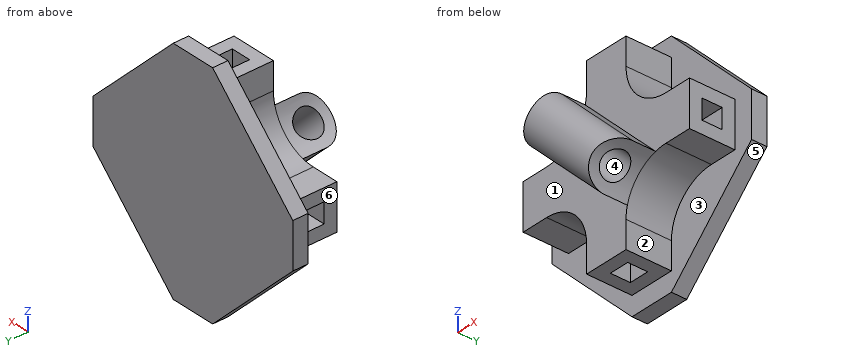
```python
from build123d import *

# Parameters (mm, degrees)
BOSS_EXTRUDE1_DEPTH                  = 7.5184
SKETCH2_W                            = 3.302
SKETCH2_H                            = 3.302
CUT_EXTRUDE1_DEPTH                   = 12.7
CIRPATTERN1_COUNT                    = 4
BOSS_EXTRUDE2_DEPTH                  = 2.54
BOSS_EXTRUDE3_REACH                  = 29.97
BOSS_EXTRUDE3_END_RADIUS             = 7.62
SKETCH6_R                            = 2.2225
BOSS_EXTRUDE3_DIRECTION_2_REACH      = 29.97
BOSS_EXTRUDE3_DIRECTION_2_END_RADIUS = 7.62


with BuildPart() as part:
    # Sketch1 → Boss-Extrude1 (new body)
    with BuildSketch(Plane(origin=(0, 0, 0), x_dir=(1, 0, 0), z_dir=(0, 1, 0))):
        with BuildLine():
            Line((3.7592, 11.3792), (3.7592, 15.875))
            Line((3.7592, 15.875), (-3.7592, 15.875))
            Line((-3.7592, 15.875), (-3.7592, 11.3792))
            ThreePointArc((-3.7592, 11.3792), (-5.991046327, 5.991046327), (-11.3792, 3.7592))
            Line((-11.3792, 3.7592), (-15.875, 3.7592))
            Line((-15.875, 3.7592), (-15.875, -3.7592))
            Line((-15.875, -3.7592), (-11.3792, -3.7592))
            ThreePointArc((-11.3792, -3.7592), (-5.991046327, -5.991046327), (-3.7592, -11.3792))
            Line((-3.7592, -11.3792), (-3.7592, -15.875))
            Line((-3.7592, -15.875), (3.7592, -15.875))
            Line((3.7592, -15.875), (3.7592, -11.3792))
            ThreePointArc((3.7592, -11.3792), (5.991046327, -5.991046327), (11.3792, -3.7592))
            Line((11.3792, -3.7592), (15.875, -3.7592))
            Line((15.875, -3.7592), (15.875, 3.7592))
            Line((15.875, 3.7592), (11.3792, 3.7592))
            ThreePointArc((11.3792, 3.7592), (5.991046327, 5.991046327), (3.7592, 11.3792))
        make_face()
    extrude(amount=-BOSS_EXTRUDE1_DEPTH)

    # Sketch2 → Cut-Extrude1 (cut)
    with BuildSketch(Plane.XY.offset(15.875)):
        with Locations((0, -3.7592)):
            Rectangle(SKETCH2_W, SKETCH2_H)
    cut_extrude1 = extrude(amount=-CUT_EXTRUDE1_DEPTH, mode=Mode.SUBTRACT)

    # CirPattern1: Cut-Extrude1 ×4 about axis
    cirpattern1_axis = Axis((0, 0, 0), (0, 1, 0))
    for i in range(1, CIRPATTERN1_COUNT):
        add(cut_extrude1.rotate(cirpattern1_axis, i * 360 / CIRPATTERN1_COUNT), mode=Mode.SUBTRACT)

    # Sketch4 → Boss-Extrude2 (add)
    with BuildSketch(Plane(origin=(0, 0, 0), x_dir=(1, 0, 0), z_dir=(0, 1, 0))):
        Polygon((3.7592, 19.05), (19.05, 3.7592), (19.05, -3.7592), (3.7592, -19.05), (-3.7592, -19.05), (-19.05, -3.7592), (-19.05, 3.7592), (-3.7592, 19.05), align=None)
    extrude(amount=BOSS_EXTRUDE2_DEPTH)

    # Boss-Extrude3: up to this cylinder (the profile starts outside it)
    boss_extrude3_end = Plane(origin=(-11.3792, -9.4234, 11.3792), z_dir=(0, 1, 0)) * Cylinder(BOSS_EXTRUDE3_END_RADIUS, 76.18, mode=Mode.PRIVATE)
    # Sketch6 → Boss-Extrude3 (add, up to the surface)
    with BuildSketch(Plane(origin=(0, 0, 0), x_dir=(0.7071067811865474, 0, 0.7071067811865477), z_dir=(-0.7071067811865477, 0, 0.7071067811865474)), mode=Mode.PRIVATE) as boss_extrude3_sk1:
        with BuildLine():
            Line((-3.81, -11.3284), (-3.81, -7.5184))
            Line((-3.81, -7.5184), (3.81, -7.5184))
            Line((3.81, -7.5184), (3.81, -11.3284))
            ThreePointArc((3.81, -11.3284), (0, -15.1384), (-3.81, -11.3284))
        make_face()
        with Locations(Location((0, -11.3284, 0), (0, 0, 180))):
            Circle(SKETCH6_R, mode=Mode.SUBTRACT)
    boss_extrude3_tool1 = extrude(boss_extrude3_sk1.sketch, amount=BOSS_EXTRUDE3_REACH, mode=Mode.PRIVATE) - boss_extrude3_end
    add(boss_extrude3_tool1.solids().sort_by_distance((-2.617877, -9.4234, -2.617877))[0])

    # Boss-Extrude3 direction 2: up to this cylinder (the profile starts outside it)
    boss_extrude3_direction_2_end = Plane(origin=(11.3792, -9.4234, -11.3792), z_dir=(0, 1, 0)) * Cylinder(BOSS_EXTRUDE3_DIRECTION_2_END_RADIUS, 76.18, mode=Mode.PRIVATE)
    # Sketch6 → Boss-Extrude3 direction 2 (add, up to the surface)
    with BuildSketch(Plane(origin=(0, 0, 0), x_dir=(0.7071067811865474, 0, 0.7071067811865477), z_dir=(-0.7071067811865477, 0, 0.7071067811865474)), mode=Mode.PRIVATE) as boss_extrude3_direction_2_sk1:
        with BuildLine():
            Line((-3.81, -11.3284), (-3.81, -7.5184))
            Line((-3.81, -7.5184), (3.81, -7.5184))
            Line((3.81, -7.5184), (3.81, -11.3284))
            ThreePointArc((3.81, -11.3284), (0, -15.1384), (-3.81, -11.3284))
        make_face()
        with Locations(Location((0, -11.3284, 0), (0, 0, 180))):
            Circle(SKETCH6_R, mode=Mode.SUBTRACT)
    boss_extrude3_direction_2_tool1 = extrude(boss_extrude3_direction_2_sk1.sketch, amount=-BOSS_EXTRUDE3_DIRECTION_2_REACH, mode=Mode.PRIVATE) - boss_extrude3_direction_2_end
    add(boss_extrude3_direction_2_tool1.solids().sort_by_distance((-2.617877, -9.4234, -2.617877))[0])


solid = part.part
```
The listing builds one solid part. Answer for the finished solid, in the listing's coordinates (mm). Face numbers are marked on the shaded views. A direction names the side the tool comes from. Coordinates: 2 decimals unless noted, no trailing zeros. Write each loop counter-clockwise with the first axis right and the second up, starting at its lowest first coordinate (ties: lowest second). Pieces come first, ordered by that corner, then holes. Notation, with made-up numbers: (71, 58.5) - (106, 58.5) arc R36 ccw to (106, 97.5) - close; hole circle Ø6 at (84.25, 5). An arc over 180 degrees is marked (long way). One line per item, written item: value.
1) Consider line 1 along Y through (x, z) = (-1, 14.5); line 2 along X through (y, z) = (-3.5, -15); line 3 along Y through (x, z) = (0, -16). Determine where each line is inside the solid, lowest interval first. Write a range as from..to.
Geometry check:
line 1: y = -7.52..-5.41, -2.11..2.54
line 2: x = -3.76..-1.65, 1.65..3.76
line 3: y = 0..2.54
2) Find section B-B (z = 15). Give the vertices of the cut face in (x, y), and give its area (3 significant figures).
Geometry check:
outline: (-7.81, 0) - (-3.76, 0) - (-3.76, -7.52) - (3.76, -7.52) - (3.76, 0) - (7.81, 0) - (7.81, 2.54) - (-7.81, 2.54) - close; hole (-1.65, -5.41) - (1.65, -5.41) - (1.65, -2.11) - (-1.65, -2.11) - close
area: 85.3 mm2
3) For a pull along Z with two mould halves and no side action, classify the marked faces 4, 5 and 6 as pulls with the +Z half, pulls with the -Z half, needs draft (parallel to the pull), parting line crosses it, or undercut.
Geometry check:
face 4: undercut
face 5: pulls with the -Z half
face 6: needs draft
4) Each of these flat-tipped pins is pushed along its axis until it touches: pin 1 Ø2.5 at (x, y) = (-12, -4) entering from +Z; pin 2 Ø2 at (y, z) = (-3.5, 12.5) entering from +X; pin 3 Ø8 at (y, z) = (-7.5, -1) entering from -X (3 decimals). Where does it stop, or does it pass through?
Geometry check:
pin 1: stops at z = 3.79
pin 2: stops at x = 3.76
pin 3: stops at x = -15.875
5) Find section D-D (y = -10.75). Give the vertices of the cut face in (x, z).
Geometry check:
outline: (-9.41, 4.02) - (4.02, -9.41) arc R7.62 cw to (4.69, -7.73) - (-7.73, 4.69) arc R7.62 cw to start; (-4.69, 7.73) - (7.73, -4.69) arc R7.62 cw to (9.41, -4.02) - (-4.02, 9.41) arc R7.62 cw to start
6) Find section C-C (x = -14). Give the vertices of the cut face in (y, z), and give its area (3 significant figures).
Geometry check:
outline: (-7.52, -3.76) - (0, -3.76) - (0, -8.81) - (2.54, -8.81) - (2.54, 8.81) - (0, 8.81) - (0, 3.76) - (-7.52, 3.76) - close; hole (-5.41, -1.65) - (-2.11, -1.65) - (-2.11, 1.65) - (-5.41, 1.65) - close
area: 90.4 mm2
7) A tool of negligible diameter and unlimited length cuts with its end or side. For the marked faces 1, 2 and 3, from which of +Z, -Z, +X, -X, +Y, -Y can it reach the whole face along a straight path? Write none if from no direction.
Geometry check:
face 1: -Z, -X, -Y
face 2: -Z, +X, -Y
face 3: -Y
